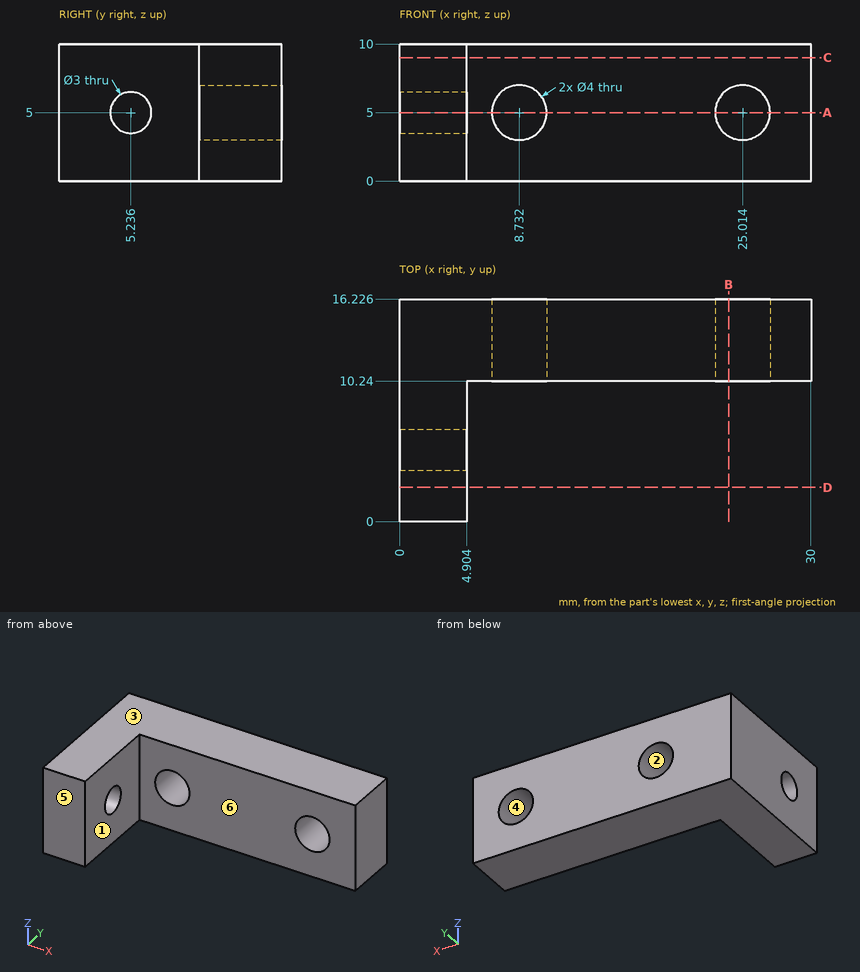
Part print with two shaded views. Sizes in mm from the minimum x, y, z corner. A direction names the side the tool comes from. Round coordinates to 2 decimals unless told otherwise and drop trailing zeros. Loops run counter-clockwise (first coordinate to the right, second up) from the corner with the lowest first, then second, coordinate; pieces in that order, holes last. Notation, with made-up numbers: M 9.5,10.5 L 23.5,10.5 A36 ccw 23.5,47.5 Z; hole C 29.5,52.25 d6. An arc over 180 degrees is marked long. Return JSON: item names as keys, results as strings. Group by question number.
(1) Drop flat-ended pins along their axis: P1, Ø6, axis at x = 7.5, y = 5, coming from the +Z side; P2, Ø2, axis at x = 18, z = 3, coming from the -Y side; P3, Ø2.5, axis at x = 25.01, z = 5, coming from the +Y side. Give the stop position or say it passes through.
(2) Saw through at B-B, the plane x = 24. List the corners of the cut face in (y, z).
(3) Saw through at C-C, the plane z = 9. List the corners of the cut face in (x, y).
(4) Wall check: probe 1 along X at (y, z) = (13.4, 5); probe 2 along X at (y, z) = (14.25, 6.25) (1 decimal); probe 3 along Y at (x, z) = (17, 7.5). Give the ranges that are in metal, low to high. Write a range as [from, to].
(5) Saw through at D-D, the plane y = 2.5. List the corners of the cut face in (x, z).
(6) Tool access for the marked faces 5 and 6: list every direction of +Z, -Z, +X, -X, +Y, -Y with a clear straight run to the whole face (end or side of a thin tool).
(7) Saw through at A-A, the plane z = 5. List the corners of the cut face in (x, y).
(8) Mould opens along X. For the marked faces 1, 2, 3 and 4 say: +X half, -X half, draft (parallel to the pull), parting line (faces both ways), or undercut.
Answer list:
{
 "1": {"P1": "z = 10", "P2": "y = 10.24", "P3": "through"},
 "2": {"outline": "M 10.24,0 L 16.23,0 L 16.23,3.28 L 10.24,3.28 Z; M 10.24,6.72 L 16.23,6.72 L 16.23,10 L 10.24,10 Z"},
 "3": {"outline": "M 0,0 L 4.9,0 L 4.9,10.24 L 30,10.24 L 30,16.23 L 0,16.23 Z"},
 "4": {"probe 1": "[0, 6.73], [10.73, 23.01], [27.01, 30]", "probe 2": "[0, 7.2], [10.3, 23.5], [26.6, 30]", "probe 3": "[10.24, 16.23]"},
 "5": {"outline": "M 0,0 L 4.9,0 L 4.9,10 L 0,10 Z"},
 "6": {"face 5": "+Z, -Z, +X, -X, -Y", "face 6": "+Z, -Z, +X, -Y"},
 "7": {"outline": "M 0,0 L 4.9,0 L 4.9,3.74 L 0,3.74 Z; M 0,6.74 L 4.9,6.74 L 4.9,10.24 L 6.73,10.24 L 6.73,16.23 L 0,16.23 Z; M 10.73,10.24 L 23.01,10.24 L 23.01,16.23 L 10.73,16.23 Z; M 27.01,10.24 L 30,10.24 L 30,16.23 L 27.01,16.23 Z"},
 "8": {"face 1": "+X half", "face 2": "undercut", "face 3": "draft", "face 4": "undercut"}
}
